The model under review builds one solid part; all positions refer to its coordinate system, in mm. A direction names the side the tool comes from. Give positions to 0.01 mm unless a question says otherwise; leave off trailing zeros. Loops run counter-clockwise (first coordinate to the right, second up) from the corner with the lowest first, then second, coordinate; pieces in that order, holes last. Notation, with made-up numbers: M 70.25,-1 L 85.25,-1 A15 ccw 85.25,8 Z; hole C 1,-35 d6. An arc over 180 degrees is marked long. One line per item, written item: value. Start each with the question number.
Q1. For pin 1 (3 mm diameter, centred on x = 10.5, z = 14, fed in from -Y); pin 2 (2 mm diameter, centred on x = -19.05, y = 0, fed in from +Z); pin 3 (1 mm diameter, centred on x = 15.5, y = 10.5, fed in from +Z); pin 4 (2 mm diameter, centred on x = 18.5, y = -13, fed in from -Z), all flat-tipped, find the tip position at first contact; note any pin that passes through.
Q2. Mouldability with a two-part tool opening along Y and no side actions: class faces 3 (the face through (19.69, 1.01, 74.95)), 4 (the face through (-19.69, -1.01, 74.95)), 5 (the face through (0, 0, 0)), 6 (the face through (-0.41, 12.04, 87.97)) as released by +Y, released by -Y, zero draft, split by the parting line, or undercut.
Q3. For faces 1 (the face through (-19, 0, 73.66)), 2 (the face through (0, 9, 100.076)), list the 3-axis set-ups (+Z, -Z, +X, -X, +Y, -Y) from which the entire face can be reached by the end or side of a thin tool; tool diameter is ignored.
Q4. We need section A-A on x = 0. Write out the cut boundary in (y, z) (3 decimals).
Q5. We need section C-C on z = 94. Write out the cut boundary in (x, y) (3 decimals), plus the area to 3 significant figures.
Q6. To check wall thickness, follow line 1 along Z through (x, y) = (-9, -2); line 2 along Z through (x, y) = (18.5, 0); line 3 along Y through (x, z) = (19.05, 75.5). State the ranges of each line that lie inside material, in increasing order. Write a range as from..to.
Q7. We need section B-B on y = 0. Write out the cut boundary in (x, z), plus the area to 3 significant figures.
Q8. We need section D-D on y = 8.89. Write out the cut boundary in (x, z) (3 decimals), plus the area to 3 significant figures.
```python
from build123d import *

# Parameters (mm, degrees)
SKETCH1_R           = 25.4
BOSS_EXTRUDE1_DEPTH = 76.2
SKETCH2_R           = 3.175
BOSS_EXTRUDE2_DEPTH = 23.876
SKETCH3_R           = 1.19681919
CUT_EXTRUDE1_DEPTH  = 2.54


with BuildPart() as part:
    # Sketch1 → Boss-Extrude1 (new body)
    with BuildSketch(Plane.XY):
        with Locations(Location((0, 0, 0), (0, 0, 180))):
            Circle(SKETCH1_R)
    extrude(amount=BOSS_EXTRUDE1_DEPTH)

    # Sketch2 → Boss-Extrude2 (add)
    with BuildSketch(Plane.XY.offset(76.2)):
        with Locations((0, 8.89)):
            Circle(SKETCH2_R)
    extrude(amount=BOSS_EXTRUDE2_DEPTH)

    # Sketch3 → Cut-Extrude1 (cut)
    with BuildSketch(Plane.XY.offset(76.2)):
        with Locations((19.05, 0)):
            Circle(SKETCH3_R)
        with Locations(Location((-19.05, 0, 0), (0, 0, 180))):
            Circle(SKETCH3_R)
    extrude(amount=-CUT_EXTRUDE1_DEPTH, mode=Mode.SUBTRACT)


solid = part.part
```
Solved:
1. pin 1: y = -23.75
1. pin 2: z = 73.66
1. pin 3: z = 76.2
1. pin 4: z = 0
2. face 3: undercut
2. face 4: undercut
2. face 5: zero draft
2. face 6: split by the parting line
3. face 1: +Z
3. face 2: +Z, +X, -X, +Y, -Y
4. outline: M -25.4,0 L 25.4,0 L 25.4,76.2 L 12.065,76.2 L 12.065,100.076 L 5.715,100.076 L 5.715,76.2 L -25.4,76.2 Z
5. outline: C 0,8.89 d6.35
5. area: 31.7 mm2
6. line 1: 0..76.2
6. line 2: 0..73.66
6. line 3: -16.8..-1.2, 1.2..16.8
7. outline: M -25.4,0 L 25.4,0 L 25.4,76.2 L 20.25,76.2 L 20.25,73.66 L 17.85,73.66 L 17.85,76.2 L -17.85,76.2 L -17.85,73.66 L -20.25,73.66 L -20.25,76.2 L -25.4,76.2 Z
7. area: 3,860 mm2
8. outline: M -23.793,0 L 23.793,0 L 23.793,76.2 L 3.175,76.2 L 3.175,100.076 L -3.175,100.076 L -3.175,76.2 L -23.793,76.2 Z
8. area: 3,780 mm2
